Build history of the part. All positions in model axes, mm. Face numbers are marked on the shaded views. A direction names the side the tool comes from. Coordinates: 2 decimals unless noted, no trailing zeros. Order: outer loops, then holes, each group sorted by start corner. A loop starts at its lowest first (then second) coordinate and runs counter-clockwise, first axis right, second up. Notation, with made-up numbers: (-29.5, 24.25) - (3.5, 24.25) arc R11 ccw to (3.5, 29.25) - close; hole circle Ø9 at (47, 57). An arc over 180 degrees is marked (long way). Answer as CSV lines item,"result". Start each with the question number.
from build123d import *
from OCP.BRepFilletAPI import BRepFilletAPI_MakeChamfer

# Parameters (mm, degrees)
SKETCH_3_R          = 5
EXTRUDE_2_DEPTH     = 9
SKETCH_4_R          = 4
EXTRUDE_3_DEPTH     = 2
SKETCH_5_R          = 5
EXTRUDE_4_DEPTH     = 9
CUT_EXTRUDE_5_REACH = 23.213
CHAMFER_2_SIZE      = 1.7
CHAMFER_2_SIZE2     = 0.981495458


with BuildPart() as part:
    # Эскиз3 → Вытянуть2 (new body)
    with BuildSketch(Plane.XY):
        Circle(SKETCH_3_R)
    extrude(amount=EXTRUDE_2_DEPTH)

    # Эскиз4 → Вытянуть3 (add)
    with BuildSketch(Plane.XY.offset(9)):
        Circle(SKETCH_4_R)
    extrude(amount=EXTRUDE_3_DEPTH)

    # Эскиз5 → Вытянуть4 (add)
    with BuildSketch(Plane.XY.offset(11)):
        Circle(SKETCH_5_R)
    extrude(amount=EXTRUDE_4_DEPTH)

    # Эскиз1 → Вытянуть5 (cut, up to next)
    with BuildSketch(Plane.XY, mode=Mode.PRIVATE) as cut_extrude_5_sk1:
        with BuildLine():
            Line((2, 1.813835715), (2, -1.813835715))
            ThreePointArc((2, -1.813835715), (-2.7, 0), (2, 1.813835715))
        make_face()
    cut_extrude_5_tool1 = extrude(cut_extrude_5_sk1.sketch, amount=CUT_EXTRUDE_5_REACH, mode=Mode.PRIVATE) & part.part
    add(cut_extrude_5_tool1.solids().sort_by_distance((-0.188014, 0, 0))[0], mode=Mode.SUBTRACT)

    # Фаска2: one chamfer whose edges measure the first distance from different faces: ONE call of the kernel's chamfer builder (chamfer() names one face for all edges)
    chamfer_2_edges_1 = [part.edges().sort_by_distance(p)[0] for p in [
        (-5, 0, 9),
    ]]
    chamfer_2_side_1 = [part.faces().sort_by_distance(p)[0] for p in [
        (-5, 0, 4.5),
    ]]
    chamfer_2_edges_2 = [part.edges().sort_by_distance(p)[0] for p in [
        (-5, 0, 11),
    ]]
    chamfer_2_side_2 = [part.faces().sort_by_distance(p)[0] for p in [
        (-5, 0, 15.5),
    ]]
    chamfer_2 = BRepFilletAPI_MakeChamfer(part.part.solid().wrapped)
    for e in chamfer_2_edges_1:
        chamfer_2.Add(CHAMFER_2_SIZE, CHAMFER_2_SIZE2, e.wrapped, chamfer_2_side_1[0].wrapped)  # the first distance lies on this face
    for e in chamfer_2_edges_2:
        chamfer_2.Add(CHAMFER_2_SIZE, CHAMFER_2_SIZE2, e.wrapped, chamfer_2_side_2[0].wrapped)  # the first distance lies on this face
    add(Compound.cast(chamfer_2.Shape()), mode=Mode.REPLACE)


solid = part.part
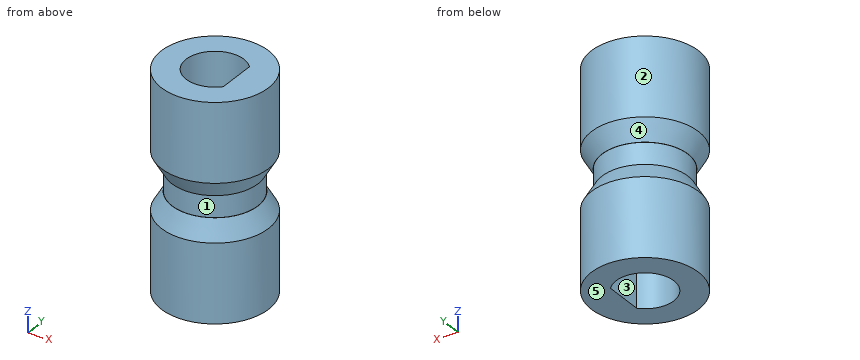
(1) Pull direction Z, two halves, no side cores. Call the marked faces 3, 4 and 5: +Z half, -Z half, draft (parallel to the pull), parting line (faces both ways), or undercut.
(2) Drop flat-ended pins along their axis: pin 1 Ø1 at (y, z) = (3.5, 17.5) entering from +X; pin 2 Ø1.1 at (y, z) = (-0.5, 9) entering from -X; pin 3 Ø6 at (y, z) = (-3, 9.5) entering from -X. Give the stop position or say it passes through.
(3) Which spindle directions (+Z, -Z, +X, -X, +Y, -Y) get a long thin tool onto all of the face, cutting with end or side? Do the marked faces 1 and 2. Say none if no direction does.
(4) Probe L1, parallel to Y at x = 0, z = 5.25; L2, parallel to Y at x = 1, z = 4.5; L3, parallel to X at y = -2.25, z = 1. List the from-to ranges inside material, lowest first. Write a range as [from, to].
(5) Band-saw the part on C-C on z = 9.75. List the corners of the cut face in (x, y), plus the area to 3 significant figures.
Filled in:
1,face 3,"draft"
1,face 4,"undercut"
1,face 5,"-Z half"
2,pin 1,"stops at x = 4"
2,pin 2,"stops at x = -4.31"
2,pin 3,"stops at x = -4.91"
3,face 1,"none"
3,face 2,"+Z, -Z"
4,L1,"y = [-5, -2.7], [2.7, 5]"
4,L2,"y = [-4.9, -2.51], [2.51, 4.9]"
4,L3,"x = [-4.47, -1.49], [1.49, 4.47]"
5,outline,"circle Ø8 at (0, 0); hole (2, -1.81) - (2, 1.81) arc R2.7 ccw (long way) to start"
5,area,"29.1 mm^2"
